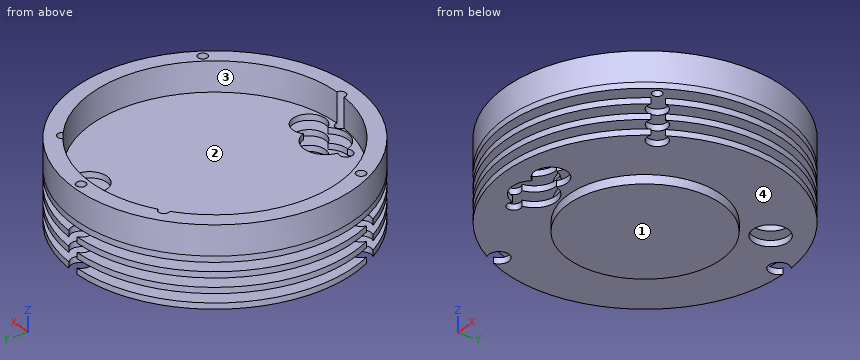
from build123d import *

# Parameters (mm, degrees)
SKETCH1_R                                           = 47.5
SKETCH1_R_2                                         = 42
BOSS_EXTRUDE1_DEPTH                                 = 10
BOSS_EXTRUDE2_START                                 = 20
SKETCH4_R                                           = 47.5
BOSS_EXTRUDE2_DEPTH                                 = 20
SKETCH5_R                                           = 47.5
SKETCH5_R_2                                         = 26
CUT_EXTRUDE1_DEPTH                                  = 3
LPATTERN1_COUNT                                     = 4
LPATTERN1_PITCH                                     = 5
CBORE_FOR_4_BINDING_HEAD_MACHINE_SCREW3_D           = 3.2639
CBORE_FOR_4_BINDING_HEAD_MACHINE_SCREW3_CBORE_D     = 6.74624
CBORE_FOR_4_BINDING_HEAD_MACHINE_SCREW3_CBORE_DEPTH = 14.4272
CIRPATTERN2_COUNT                                   = 3
SKETCH16_R                                          = 1.75
CUT_EXTRUDE2_DEPTH                                  = 12
CIRPATTERN3_COUNT                                   = 5
SKETCH21_R                                          = 6
CUT_EXTRUDE5_DEPTH                                  = 20
SKETCH22_R                                          = 7.4
CUT_EXTRUDE6_DEPTH                                  = 22
SKETCH23_R                                          = 5.5
CUT_EXTRUDE7_DEPTH                                  = 22
SKETCH24_R                                          = 2.2
CUT_EXTRUDE8_DEPTH                                  = 22


with BuildPart() as part:
    # Sketch1 → Boss-Extrude1 (new body)
    with BuildSketch(Plane.XY):
        Circle(SKETCH1_R)
        Circle(SKETCH1_R_2, mode=Mode.SUBTRACT)
    extrude(amount=BOSS_EXTRUDE1_DEPTH)

    # Sketch4 → Boss-Extrude2 (add)
    with BuildSketch(Plane(origin=(0, 0, 0), x_dir=(-1, 0, 0), z_dir=(0, 0, -1)).offset(BOSS_EXTRUDE2_START)):
        Circle(SKETCH4_R)
    extrude(amount=-BOSS_EXTRUDE2_DEPTH)

    # Sketch5 → Cut-Extrude1 (cut)
    with BuildSketch(Plane(origin=(0, 0, -20), x_dir=(-1, 0, 0), z_dir=(0, 0, -1))):
        Circle(SKETCH5_R)
        Circle(SKETCH5_R_2, mode=Mode.SUBTRACT)
    cut_extrude1 = extrude(amount=-CUT_EXTRUDE1_DEPTH, mode=Mode.SUBTRACT)

    # LPattern1: Cut-Extrude1 ×4
    with Locations(*[(0, 0, i * LPATTERN1_PITCH) for i in range(1, LPATTERN1_COUNT)]):
        add(cut_extrude1, mode=Mode.SUBTRACT)

    # CBORE for #4 Binding Head Machine Screw3 (through all)
    with Locations(Plane(origin=(0, 0, -17), x_dir=(-1, 0, 0), z_dir=(0, 0, -1))):
        with Locations((0, 44.75)):
            cbore_for_4_binding_head_machine_screw3 = CounterBoreHole(CBORE_FOR_4_BINDING_HEAD_MACHINE_SCREW3_D / 2, CBORE_FOR_4_BINDING_HEAD_MACHINE_SCREW3_CBORE_D / 2, CBORE_FOR_4_BINDING_HEAD_MACHINE_SCREW3_CBORE_DEPTH)

    # CirPattern2: CBORE for #4 Binding Head Machine Screw3 ×3 about axis
    cirpattern2_axis = Axis((0, 0, 0), (0, 0, 1))
    for i in range(1, CIRPATTERN2_COUNT):
        add(cbore_for_4_binding_head_machine_screw3.rotate(cirpattern2_axis, i * 360 / CIRPATTERN2_COUNT), mode=Mode.SUBTRACT)

    # Sketch16 → Cut-Extrude2 (cut)
    with BuildSketch(Plane.XY.offset(10)):
        with Locations((0, -42)):
            Circle(SKETCH16_R)
    cut_extrude2 = extrude(amount=-CUT_EXTRUDE2_DEPTH, mode=Mode.SUBTRACT)

    # CirPattern3: Cut-Extrude2 ×5 about axis, 2 skipped
    cirpattern3_axis = Axis((0, 0, 10), (0, 0, -1))
    add([cut_extrude2.rotate(cirpattern3_axis, i * 360 / CIRPATTERN3_COUNT) for i in range(1, CIRPATTERN3_COUNT) if i not in (1, 4)], mode=Mode.SUBTRACT)

    # Sketch21 → Cut-Extrude5 (cut)
    with BuildSketch(Plane(origin=(0, 0, -20), x_dir=(-1, 0, 0), z_dir=(0, 0, -1))):
        with Locations((-13.43425834, 32.776896042)):
            Circle(SKETCH21_R)
    extrude(amount=-CUT_EXTRUDE5_DEPTH, mode=Mode.SUBTRACT)

    # Sketch22 → Cut-Extrude6 (cut)
    with BuildSketch(Plane(origin=(0, 0, -20), x_dir=(-1, 0, 0), z_dir=(0, 0, -1))):
        with Locations((4.637001489, -33.917803127)):
            Circle(SKETCH22_R)
    extrude(amount=-CUT_EXTRUDE6_DEPTH, mode=Mode.SUBTRACT)

    # Sketch23 → Cut-Extrude7 (cut)
    with BuildSketch(Plane(origin=(0, 0, -20), x_dir=(-1, 0, 0), z_dir=(0, 0, -1))):
        with Locations((-5.614995734, -35.295003963)):
            Circle(SKETCH23_R)
    extrude(amount=-CUT_EXTRUDE7_DEPTH, mode=Mode.SUBTRACT)

    # Sketch24 → Cut-Extrude8 (cut)
    with BuildSketch(Plane(origin=(0, 0, -20), x_dir=(-1, 0, 0), z_dir=(0, 0, -1))):
        with Locations((13.226831653, -34.820080994)):
            Circle(SKETCH24_R)
    extrude(amount=-CUT_EXTRUDE8_DEPTH, mode=Mode.SUBTRACT)


solid = part.part
The listing builds one solid part. Answer for the finished solid, in the listing's coordinates (mm). Face numbers are marked on the shaded views. A direction names the side the tool comes from. Round coordinates to 2 decimals unless told otherwise and drop trailing zeros. Write each loop counter-clockwise with the first axis right and the second up, starting at its lowest first coordinate (ties: lowest second). Pieces come first, ordered by that corner, then holes. Notation, with made-up numbers: (20, 80) - (60, 80) arc R9 cw to (60, 89) - close; hole circle Ø7 at (-35.5, 56.5). An arc over 180 degrees is marked (long way). Use a Markdown table: item, result. Add a question column.
1. The part is cut by section C-C (x = 34). Write down the section's boundary in (y, z), and give its area (3 significant figures).
2. The part is cut by section B-B (y = 44.75). Give the number of separate pieces and of enclosed holes in the cut face, and give its area (3 significant figures).
3. Flat-ended cylindrical pins translate along their axes: P1, Ø1.5, axis at x = -37.5, z = 5.5, coming from the -Y side; P2, Ø5, axis at x = -13.23, y = -34.82, coming from the +Z side; P3, Ø5.5, axis at x = -38.75, y = -22.37, coming from the -Z side. Find the tip coordinate at first contact, or state that the pin passes through.
4. A tool of negligible diameter and unlimited length cuts with its end or side. For the marked faces 1 and 2, from which of +Z, -Z, +X, -X, +Y, -Y can it reach the whole face along a straight path? Write none if from no direction.
5. For a pull along Y with two mould halves and no side action, classify the marked faces 3 and 4 as +Y half, -Y half, draft (parallel to the pull), parting line (faces both ways), or undercut.
6. The part is cut by section A-A (z = 4.75). Write down the section's boundary in (x, y) (3 decimals).
7. Consider line 1 (Z direction, x = -27, y = -34.5); line 2 (Z direction, x = -26, y = 33.5); line 3 (Z direction, x = -29.5, y = -7). Determine where each line is inside the solid, lowest interval first.
Reported:
| question | item | result |
|---|---|---|
| 1 | outline | (-33.17, -17) - (33.17, -17) - (33.17, -15) - (-33.17, -15) - close; (-33.17, -12) - (33.17, -12) - (33.17, -10) - (-33.17, -10) - close; (-33.17, -7) - (33.17, -7) - (33.17, -5) - (-33.17, -5) - close; (-33.17, -2) - (33.17, -2) - (33.17, 10) - (24.66, 10) - (24.66, 0) - (-24.66, 0) - (-24.66, 10) - (-33.17, 10) - close |
| 1 | area | 701 mm^2 |
| 2 | separate pieces | 8 |
| 2 | enclosed holes | 0 |
| 2 | area | 494 mm^2 |
| 3 | P1 | y = -30.09 |
| 3 | P2 | z = 0 |
| 3 | P3 | z = -2 |
| 4 | face 1 | -Z, +X, -X, +Y, -Y |
| 4 | face 2 | +Z |
| 5 | face 3 | undercut |
| 5 | face 4 | draft |
| 6 | outline | circle Ø95 at (0, 0); hole circle Ø3.264 at (-38.755, -22.375); hole (-26.081, 32.921) arc R42 ccw to (-1.75, -41.964) arc R1.75 ccw (long way) to (1.75, -41.964) arc R42 ccw to (26.081, 32.921) arc R1.75 ccw (long way) to (23.25, 34.978) arc R42 ccw to (-23.25, 34.978) arc R1.75 ccw (long way) to start; hole circle Ø3.264 at (0, 44.75); hole circle Ø3.264 at (38.755, -22.375) |
| 7 | line 1 | -17 to -15, -12 to -10, -7 to -5, -2 to 10 |
| 7 | line 2 | -17 to -15, -12 to -10, -7 to -5 |
| 7 | line 3 | -17 to -15, -12 to -10, -7 to -5, -2 to 0 |
